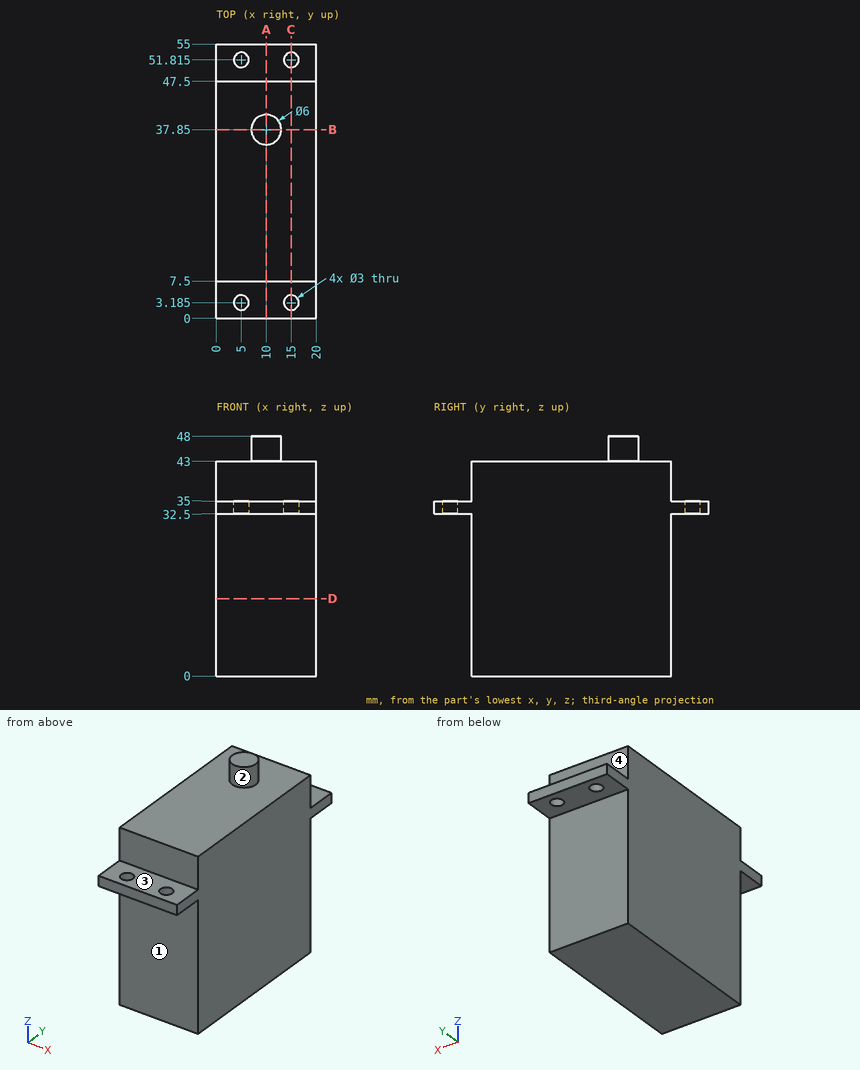
For this review, use the dimensioned drawing (mm, ordinates from the lowest corner) and the shaded views. A direction names the side the tool comes from. Give positions to 0.01 mm unless a question says otherwise; leave off trailing zeros. Order: outer loops, then holes, each group sorted by start corner. A loop starts at its lowest first (then second) coordinate and runs counter-clockwise, first axis right, second up. Notation, with made-up numbers: (44, -34.75) - (48, -34.75) arc R17 ccw to (48, -22.75) - close; hole circle Ø4 at (33.25, 15). An arc over 180 degrees is marked (long way). Use a Markdown table: item, result. Add a question column.
(1) Add section A-A on x = 10. Give the boundary of the cut face in (y, z), then the cut area to 3 significant figures.
(2) Add section D-D on z = 15.5. Give the boundary of the cut face in (x, y), then the cut area to 3 significant figures.
(3) Add section B-B on y = 37.85. Give the boundary of the cut face in (x, z).
(4) Machinability: for the marked faces 1, 2, 3 and 4, which of the approach directions +Z, -Z, +X, -X, +Y, -Y give a long, thin tool a straight path to every point of the face, cutting with its end or side? Answer none if there is none.
(5) Add section C-C on x = 15. Give the boundary of the cut face in (y, z) (3 decimals).
(6) Wall thickness on probe 1 along Y at (x, z) = (15, 34.15) (3 decimals); probe 2 along Y at (x, z) = (6, 22.5); probe 3 along Z at (x, y) = (11, 29.5): over which ranges is each line inside the solid? List them lowest first. Write a range as [from, to].
(7) Clearance check with flat-ended pins moving along their axes: P1, Ø1.5, axis at x = 7.5, z = 32, coming from the +Y side; P2, Ø4, axis at x = 15, y = 3.185, coming from the -Z side; P3, Ø6, axis at x = 6.5, y = 4, coming from the +Z side; P4, Ø1.8, axis at x = 5, y = 3.185, coming from the -Z side. State where each tip first meets the part, or that it passes through.
Report:
| question | item | result |
|---|---|---|
| 1 | outline | (0, 32.5) - (7.5, 32.5) - (7.5, 0) - (47.5, 0) - (47.5, 32.5) - (55, 32.5) - (55, 35) - (47.5, 35) - (47.5, 43) - (40.85, 43) - (40.85, 48) - (34.85, 48) - (34.85, 43) - (7.5, 43) - (7.5, 35) - (0, 35) - close |
| 1 | area | 1,790 mm² |
| 2 | outline | (0, 7.5) - (20, 7.5) - (20, 47.5) - (0, 47.5) - close |
| 2 | area | 800 mm² |
| 3 | outline | (0, 0) - (20, 0) - (20, 43) - (13, 43) - (13, 48) - (7, 48) - (7, 43) - (0, 43) - close |
| 4 | face 1 | -Z, +X, -X, -Y |
| 4 | face 2 | +Z |
| 4 | face 3 | +Z, +X, -X, -Y |
| 4 | face 4 | +Z, +X, -X, +Y |
| 5 | outline | (0, 32.5) - (1.685, 32.5) - (1.685, 35) - (0, 35) - close; (4.685, 32.5) - (7.5, 32.5) - (7.5, 0) - (47.5, 0) - (47.5, 32.5) - (50.315, 32.5) - (50.315, 35) - (47.5, 35) - (47.5, 43) - (7.5, 43) - (7.5, 35) - (4.685, 35) - close; (53.315, 32.5) - (55, 32.5) - (55, 35) - (53.315, 35) - close |
| 6 | probe 1 | y = [0, 1.685], [4.685, 50.315], [53.315, 55] |
| 6 | probe 2 | y = [7.5, 47.5] |
| 6 | probe 3 | z = [0, 43] |
| 7 | P1 | stops at y = 55 |
| 7 | P2 | stops at z = 32.5 |
| 7 | P3 | stops at z = 35 |
| 7 | P4 | passes through |
